Check sheet for the drawn part. Datum: minimum x, y, z corner. Units: mm. A direction names the side the tool comes from. Give positions to 0.01 mm unless a question says otherwise; leave off trailing zeros. Order: outer loops, then holes, each group sorted by start corner. A loop starts at its lowest first (then second) coordinate and runs counter-clockwise, first axis right, second up. Notation, with made-up numbers: (34.25, 54) - (53.25, 54) arc R20 cw to (53.25, 75) - close; hole circle Ø4 at (8, -38). An arc over 180 degrees is marked (long way). Answer as a JSON object with one key per item and string values. Group by question number.
(1) Section check C-C (z = 27). Record the boundary of the cut face in (x, y), then the cut area to 3 significant figures.
(2) Thickness scan on line 1 (Y direction, x = 7, z = 21); line 2 (Y direction, x = 26, z = 14.5); line 3 (Z direction, x = 13, y = 17.75). Record the ranges inside material, lowest first.
(3) Access from +Z, -Z, +X, -X, +Y, -Y to the whole of each face (thin tool, end or side, straight path). Record for the marked faces 5, 6 and 7.
(4) Depth check by flat-ended pin: pin 1 Ø2 at (x, z) = (15.5, 17.5) entering from -Y; pin 2 Ø4 at (y, z) = (4, 18) entering from +X; pin 3 Ø3 at (y, z) = (7.5, 14) entering from +X. Enter the tip coordinate at first touch or a pass-through.
(5) Section check A-A (z = 23). Record the boundary of the cut face in (x, y).
(6) Section check B-B (x = 8). Record the boundary of the cut face in (y, z), then the cut area to 3 significant figures.
(7) Mould release check, pull along Y, two halves, no side actions. Record for the marked faces 1, 2, 3 and 4: +Y half, -Y half, draft (parallel to the pull), parting line (faces both ways), or undercut.
(8) Section check D-D (y = 9.5). Record the boundary of the cut face in (x, z).
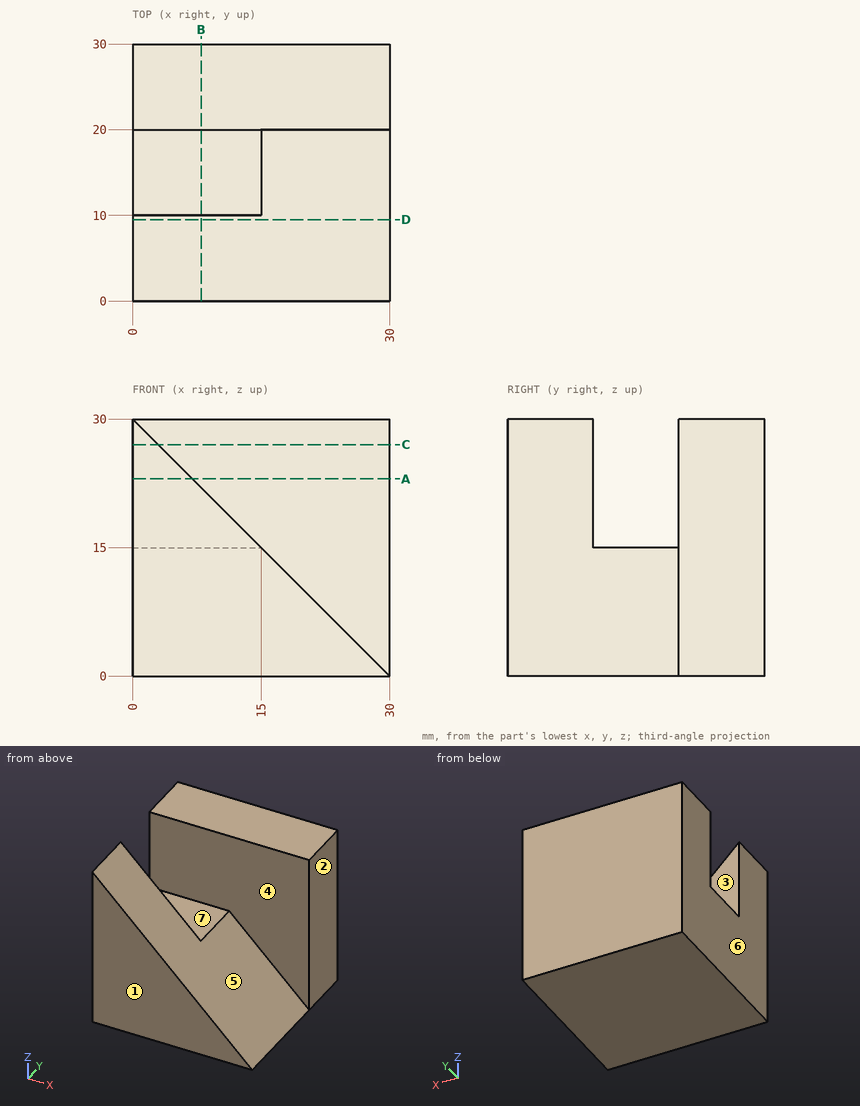
Solutions:
{
 "1": {"outline": "(0, 0) - (3, 0) - (3, 10) - (0, 10) - close; (0, 20) - (30, 20) - (30, 30) - (0, 30) - close", "area": "330 mm2"},
 "2": {"line 1": "y = 0 to 10, 20 to 30", "line 2": "y = 20 to 30", "line 3": "z = 0 to 15"},
 "3": {"face 5": "+Z, +X, -Y", "face 6": "+Z, -Z, -X, +Y, -Y", "face 7": "+Z, +X, -X"},
 "4": {"pin 1": "stops at y = 20", "pin 2": "stops at x = 14", "pin 3": "stops at x = 17.5"},
 "5": {"outline": "(0, 0) - (7, 0) - (7, 10) - (0, 10) - close; (0, 20) - (30, 20) - (30, 30) - (0, 30) - close"},
 "6": {"outline": "(0, 0) - (30, 0) - (30, 30) - (20, 30) - (20, 15) - (10, 15) - (10, 22) - (0, 22) - close", "area": "670 mm2"},
 "7": {"face 1": "-Y half", "face 2": "draft", "face 3": "undercut", "face 4": "undercut"},
 "8": {"outline": "(0, 0) - (30, 0) - (0, 30) - close"}
}
